from build123d import *

# Parameters (mm, degrees)
F1_DEPTH = 31.75
F3_DEPTH = 12.7
F5_DEPTH = 19.051


with BuildPart() as f1:
    # F0 (on Front) → F1 (new body)
    with BuildSketch(Plane.XZ):
        Polygon((50.8, 31.75), (0, 32.2926561947), (0, 0), (50.8, 0), align=None)
    extrude(amount=F1_DEPTH)

    # F2 (on face) → F3 (cut)
    with BuildSketch(Plane.XZ.offset(31.75)):
        Polygon((50.8, 31.75), (19.2072158541, 32.0874807091), (50.8, 0), align=None)
    extrude(amount=-F3_DEPTH, mode=Mode.SUBTRACT)

    # F4 (on face) → F5 (cut, through all)
    with BuildSketch(Plane.XZ.offset(19.05)):
        Polygon((32.0955355752, 18.997348845), (50.8, 18.997348845), (50.8, 31.75), (19.2072158541, 32.0874807091), align=None)
    extrude(amount=-F5_DEPTH, mode=Mode.SUBTRACT)


solid = f1.part
For this review, take the finished solid that the model builds, in its own axes (mm). A direction names the side the tool comes from. Round coordinates to 2 decimals unless told otherwise and drop trailing zeros. Write each loop counter-clockwise with the first axis right and the second up, starting at its lowest first coordinate (ties: lowest second). Pieces come first, ordered by that corner, then holes. Notation, with made-up numbers: M -6,53 L 32,53 A23 ccw 32,90 Z; hole C 1,-27 d6. An arc over 180 degrees is marked long. Write item = value, one per line. Start each with the question number.
(1) For line 1 along Z through (x, y) = (39.5, -18); line 2 along X through (y, z) = (-25, 28); line 3 along Z through (x, y) = (25.5, -7.5), list the stretches that pass through material, from the lowest coordinate up.
(2) We need section B-B (z = 9.5). Give the boundary of the cut face in (x, y), then the cut area to 3 significant figures.
(3) Clearance check with flat-ended pins moving along their axes: pin 1 Ø4 at (x, y) = (33, -8.5) entering from +Z; pin 2 Ø4 at (y, z) = (-12, 27) entering from +X; pin 3 Ø5 at (x, z) = (41.5, 15) entering from -Y. State where each tip first meets the part, or that it passes through.
(4) We need section C-C (x = 28.5). Give the boundary of the cut face in (y, z), then the cut area to 3 significant figures.
(5) For faces 1 (the face through (45, -19.05, 14)), 2 (the face through (50.8, -9, 9)), 3 (the face through (41, -10, 18.997)), list the 3-axis set-ups (+Z, -Z, +X, -X, +Y, -Y) from which the entire face can be reached by the end or side of a thin tool; tool diameter is ignored.
(6) We need section D-D (y = -25.5). Give the boundary of the cut face in (x, z), then the cut area to 3 significant figures.
(7) We need section A-A (y = -4). Give the boundary of the cut face in (x, z).
Results found:
q1.line_1 = 0 to 19
q1.line_2 = 0 to 23.23
q1.line_3 = 0 to 25.7
q2.outline = M 0,-31.75 L 41.45,-31.75 L 41.45,-19.05 L 50.8,-19.05 L 50.8,0 L 0,0 Z
q2.area = 1,490 mm²
q3.pin_1 = 20.11
q3.pin_2 = 26.19
q3.pin_3 = -19.05
q4.outline = M -31.75,0 L 0,0 L 0,22.65 L -31.75,22.65 Z
q4.area = 719 mm²
q5.face_1 = +Z, +X, -Y
q5.face_2 = +Z, -Z, +X, +Y, -Y
q5.face_3 = +Z, +X, +Y, -Y
q6.outline = M 0,0 L 50.8,0 L 19.21,32.09 L 0,32.29 Z
q6.area = 1,130 mm²
q7.outline = M 0,0 L 50.8,0 L 50.8,19 L 32.1,19 L 19.21,32.09 L 0,32.29 Z
